Design review of the part built by this model. Coordinates are the model's own, in mm. A direction names the side the tool comes from. Round coordinates to 2 decimals unless told otherwise and drop trailing zeros. Loops run counter-clockwise (first coordinate to the right, second up) from the corner with the lowest first, then second, coordinate; pieces in that order, holes last. Notation, with made-up numbers: (-1, 49) - (26, 49) arc R26 ccw to (26, 88) - close; hole circle Ø3 at (16, 37.25). An arc over 180 degrees is marked (long way). Use one line per item in the form item = value. Start each with the question number.
(1) Machinability: for faces 4 (the flat face through (3, 0, 0)), 5 (the flat face through (3, -0.8, 5)), 6 (the flat face through (3, -0.8, -5)), which of the approach directions +Z, -Z, +X, -X, +Y, -Y give a long, thin tool a straight path to every point of the face, cutting with its end or side? Answer none if there is none.
(2) For pin 1 (5.5 mm diameter, centred on x = 0, z = 0, fed in from -Y); pin 2 (0.9 mm diameter, centred on x = 1.5, z = 4.5, fed in from +Y); pin 3 (0.9 mm diameter, centred on x = 7, y = -0.5, fed in from +Z), all flat-tipped, find the tip position at first contact; note any pin that passes through.
(3) The part is to be moulded in two halves that separate along Z. For faces 1 (the cylindrical face through (-2.003, -3.448, -0.631)), 2 (the flat face through (11, -3, 0)), 3 (the flat face through (2.9, -5.5, 6.3)), say which applies: released by +Z, released by -Z, zero draft, split by the parting line, or undercut.
(4) Wall thickness on probe 1 along Z at (x, y) = (0, -3.75); probe 2 along Z at (x, y) = (7, -6.7); probe 3 along Z at (x, y) = (7, -6.65): over which ranges is each line inside the solid? List them lowest first. Write a range as [from, to].
(5) We need section D-D, the plane y = -1.5. Write out the cut boundary in (x, z), then the cut area to 3 significant figures.
(6) We need section A-A, the plane x = 0. Write out the cut boundary in (y, z), then the cut area to 3 significant figures.
(7) We need section B-B, the plane z = 0. Write out the cut boundary in (x, y), then the cut area to 3 significant figures.
(8) We need section C-C, the plane x = 7. Write out the cut boundary in (y, z), then the cut area to 3 significant figures.
from build123d import *

# Parameters (mm, degrees)
BOSS_EXTRUDE1_DEPTH = 16
FILLET1_R           = 1
FILLET2_R           = 0.5
SKETCH2_W           = 2.35
SKETCH2_H           = 0.2
TAPPED_HOLE1_D      = 4.2


with BuildPart() as part:
    # Sketch1 → Boss-Extrude1 (new body)
    with BuildSketch(Plane(origin=(-5, 0, 0), x_dir=(0, 0, -1), z_dir=(1, 0, 0))):
        Polygon((3.9, 0), (-3.9, 0), (-3.9, -0.8), (-7.5, -0.8), (-7.5, -4.3), (-5, -6.8), (5, -6.8), (7.5, -4.3), (7.5, -0.8), (3.9, -0.8), align=None)
    extrude(amount=BOSS_EXTRUDE1_DEPTH)

    # Fillet1
    fillet1_edges = [part.edges().sort_by_distance(p)[0] for p in [
        (3, -6.8, -5),
        (3, -6.8, 5),
    ]]
    fillet(fillet1_edges, radius=FILLET1_R)

    # Fillet2
    fillet2_edges = [part.edges().sort_by_distance(p)[0] for p in [
        (3, -0.8, 7.5),
        (3, -0.8, -7.5),
        (3, -4.3, -7.5),
        (3, -4.3, 7.5),
    ]]
    fillet(fillet2_edges, radius=FILLET2_R)

    # Sketch2 → Cut-Revolve1 (revolve, cut)
    with BuildSketch(Plane(origin=(7, 0, 0), x_dir=(0, 0, -1), z_dir=(1, 0, 0)), mode=Mode.PRIVATE) as cut_revolve1_sk:
        with Locations((1.175, -6.7)):
            Rectangle(SKETCH2_W, SKETCH2_H)
    revolve(cut_revolve1_sk.sketch.rotate(Axis((7, 1.665548573, 0), (0, -1, 0)), 180), axis=Axis((7, 1.665548573, 0), (0, -1, 0)), mode=Mode.SUBTRACT)

    # Sketch3 → Revolve1 (revolve)
    with BuildSketch(Plane(origin=(7, 0, 0), x_dir=(0, 0, -1), z_dir=(1, 0, 0)), mode=Mode.PRIVATE) as revolve1_sk:
        with BuildLine():
            Line((1.989974874, -6.6), (0, -6.6))
            Line((0, -6.6), (0, -7.8))
            ThreePointArc((0, -7.8), (1.161895004, -7.476784887), (1.989974874, -6.6))
        make_face()
    revolve(revolve1_sk.sketch.rotate(Axis((7, 0, 0), (0, -1, 0)), 180), axis=Axis((7, 0, 0), (0, -1, 0)))

    # Tapped Hole1 (through all)
    with Locations(Plane(origin=(0, 0, 0), x_dir=(1, 0, 0), z_dir=(0, 1, 0))):
        with Locations((0, 0)):
            Hole(TAPPED_HOLE1_D / 2)


solid = part.part
Data:
q1.face_4 = +Z, -Z, +X, -X, +Y
q1.face_5 = +Z, +X, -X, +Y
q1.face_6 = -Z, +X, -X, +Y
q2.pin_1 = -6.8
q2.pin_2 = -0.8
q2.pin_3 = 7.36
q3.face_1 = undercut
q3.face_2 = zero draft
q3.face_3 = released by +Z
q4.probe_1 = [-7.5, -2.1], [2.1, 7.5]
q4.probe_2 = [-5.02, -2.35], [-1.93, 1.93], [2.35, 5.02]
q4.probe_3 = [-5.11, -2.35], [-1.96, 1.96], [2.35, 5.11]
q5.outline = (-5, -7.5) - (11, -7.5) - (11, 7.5) - (-5, 7.5) - close; hole circle Ø4.2 at (0, 0)
q5.area = 226 mm^2
q6.outline = (-6.8, -4.59) arc R1 ccw to (-6.51, -5.29) - (-4.45, -7.35) arc R0.5 ccw to (-4.09, -7.5) - (-1.3, -7.5) arc R0.5 ccw to (-0.8, -7) - (-0.8, -3.9) - (0, -3.9) - (0, -2.1) - (-6.8, -2.1) - close; (-6.8, 2.1) - (0, 2.1) - (0, 3.9) - (-0.8, 3.9) - (-0.8, 7) arc R0.5 ccw to (-1.3, 7.5) - (-4.09, 7.5) arc R0.5 ccw to (-4.45, 7.35) - (-6.51, 5.29) arc R1 ccw to (-6.8, 4.59) - close
q6.area = 61.3 mm^2
q7.outline = (-5, -6.8) - (-2.1, -6.8) - (-2.1, 0) - (-5, 0) - close; (2.1, -6.8) - (4.65, -6.8) - (4.65, -6.6) - (5.01, -6.6) arc R2.25 ccw to (8.99, -6.6) - (9.35, -6.6) - (9.35, -6.8) - (11, -6.8) - (11, 0) - (2.1, 0) - close
q7.area = 82.7 mm^2
q8.outline = (-6.8, -4.59) arc R1 ccw to (-6.51, -5.29) - (-4.45, -7.35) arc R0.5 ccw to (-4.09, -7.5) - (-1.3, -7.5) arc R0.5 ccw to (-0.8, -7) - (-0.8, -3.9) - (0, -3.9) - (0, 3.9) - (-0.8, 3.9) - (-0.8, 7) arc R0.5 ccw to (-1.3, 7.5) - (-4.09, 7.5) arc R0.5 ccw to (-4.45, 7.35) - (-6.51, 5.29) arc R1 ccw to (-6.8, 4.59) - (-6.8, 2.35) - (-6.6, 2.35) - (-6.6, 1.99) arc R2.25 ccw to (-6.6, -1.99) - (-6.6, -2.35) - (-6.8, -2.35) - close
q8.area = 92.3 mm^2
